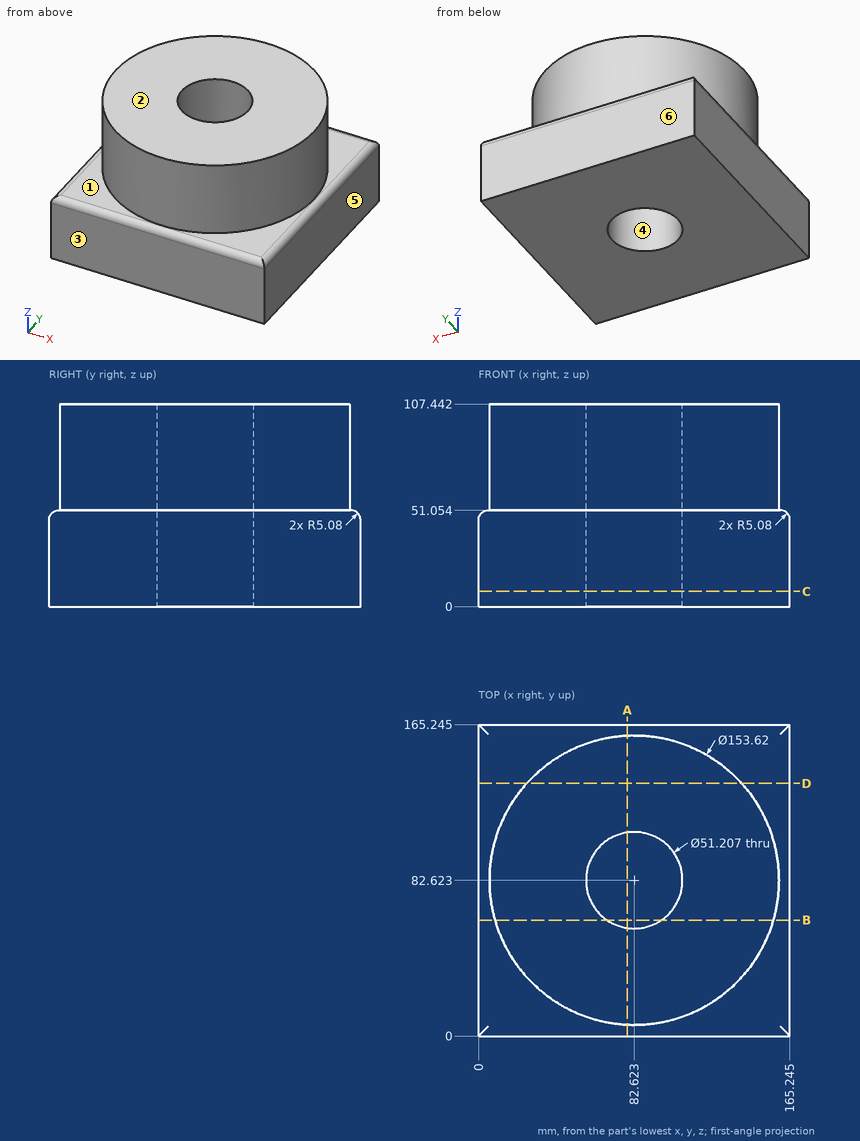
Can you work these out from the drawing? Everything is in mm from the part's minimum corner. A direction names the side the tool comes from. Round coordinates to 2 decimals unless told otherwise and drop trailing zeros. Order: outer loops, then holes, each group sorted by start corner. A loop starts at its lowest first (then second) coordinate and runs counter-clockwise, first axis right, second up.
(1) We'd pull the mould along Y, two halves only. Please class the marked faces 3, 4, 5 and 6: +Y half, -Y half, draft (parallel to the pull), parting line (faces both ways), or undercut.
Results are:
face 3: -Y half
face 4: undercut
face 5: draft
face 6: +Y half
(2) If we section it at D-D (y = 134): Please give me the cut outline in (x, z) (1 decimal), plus the area to 3 significant figures.
Results are:
outline: (0, 0) - (165.2, 0) - (165.2, 46) arc R5.1 ccw to (160.2, 51.1) - (139.7, 51.1) - (139.7, 107.4) - (25.5, 107.4) - (25.5, 51.1) - (5.1, 51.1) arc R5.1 ccw to (0, 46) - close
area: 14,900 mm2
(3) On a 3-axis mill with a long thin cutter (end or side, diameter ignored), from which of +Z, -Z, +X, -X, +Y, -Y can I reach the whole of each face in a straight line? I mean the marked faces 1 and 2. Say none if no direction works.
Results are:
face 1: +Z
face 2: +Z, +X, -X, +Y, -Y
(4) I'm going to push flat-ended pins straight in: pin 1 (8 mm diameter, centred on y = 38, z = 81.5, fed in from +X); pin 2 (2 mm diameter, centred on x = 133.5, z = 84.5, fed in from +Y) (1 decimal); pin 3 (1.5 mm diameter, centred on x = 41, z = 59, fed in from +Y) (1 decimal). Where does each tip first touch, or does it pass through?
Results are:
pin 1: stops at x = 147.81
pin 2: stops at y = 141
pin 3: stops at y = 147.7
(5) If I drill on L1, parallel to Z at x = 35, y = 158; L2, parallel to X at y = 94.5, z = 53.5 (1 decimal); L3, parallel to X at y = 86.5, z = 96 (1 decimal), over which ranges is the centre line in solid material (lowest first)?
Results are:
L1: z = 0 to 51.05
L2: x = 6.7 to 59.9, 105.3 to 158.5
L3: x = 5.9 to 57.3, 107.9 to 159.3
(6) If we section it at A-A (x = 79): Please give me the cut outline in (y, z) (1 decimal).
Results are:
outline: (0, 0) - (57.3, 0) - (57.3, 107.4) - (5.9, 107.4) - (5.9, 51.1) - (5.1, 51.1) arc R5.1 ccw to (0, 46) - close; (108, 0) - (165.2, 0) - (165.2, 46) arc R5.1 ccw to (160.2, 51.1) - (159.3, 51.1) - (159.3, 107.4) - (108, 107.4) - close
(7) If we section it at B-B (y = 61.5): Please give me the cut outline in (x, z) (1 decimal), plus the area to 3 significant figures.
Results are:
outline: (0, 0) - (68.2, 0) - (68.2, 107.4) - (8.8, 107.4) - (8.8, 51.1) - (5.1, 51.1) arc R5.1 ccw to (0, 46) - close; (97.1, 0) - (165.2, 0) - (165.2, 46) arc R5.1 ccw to (160.2, 51.1) - (156.5, 51.1) - (156.5, 107.4) - (97.1, 107.4) - close
area: 13,600 mm2
(8) If we section it at C-C (z = 8): Please give me the cut outline in (x, y) (1 decimal), plus the area to 3 significant figures.
Results are:
outline: (0, 0) - (165.2, 0) - (165.2, 165.2) - (0, 165.2) - close; hole circle Ø51.2 at (82.6, 82.6)
area: 25,200 mm2
